Geometry: final body of the model. Coordinates: model frame, mm. A direction names the side the tool comes from. Round coordinates to 2 decimals unless told otherwise and drop trailing zeros. Write each loop counter-clockwise with the first axis right and the second up, starting at its lowest first coordinate (ties: lowest second). Pieces come first, ordered by that corner, then holes. Notation, with made-up numbers: M -15,-20.5 L 17,-20.5 A22 cw 17,-11.5 Z; hole C 62.25,87.5 d5. An arc over 180 degrees is marked long. Use one line per item in the form item = value. Start each with the question number.
Item 1: Section query A-A (z = 1.4). Return loops of the section in (x, y).
Item 2: Pin query (flat end, axial travel): pin 1 Ø2 at (x, y) = (5, -2.5) entering from +Z. Return the tip coordinate at first contact, or that it passes through.
Item 3: Section query C-C (x = 10). Return loops of the section in (y, z).
Item 4: Ray query, probe 1 along X at (y, z) = (0.25, 0.45); probe 2 along X at (y, z) = (-0.25, 1.35); probe 3 along Y at (x, z) = (22.5, 1.05). Return the intervals inside material, ascending.
Item 5: Pull-direction query (Y, two-part tool) for faces 1 (the flat face through (31, -1, 2)), 2 (the cylindrical face through (26.92, -0.4, 0.99)), 3 (the cylindrical face through (12.888, -0.368, 0.597)), 4 (the cylindrical face through (-0.92, -0.4, 1.01)); classes: pulls with the +Y half, pulls with the -Y half, needs draft (parallel to the pull), parting line crosses it, or undercut.
Item 6: Reachability of faces 5 (the cylindrical face through (23.465, -0.301, 1.715)), 6 (the cylindrical face through (23.535, -1.715, 1.699)), 7 (the cylindrical face through (2.465, -1.699, 0.285)) from +Z, -Z, +X, -X, +Y, -Y: full face, straight path, thin tool, end or side. Return the list, or none.
from build123d import *

# Parameters (mm, degrees)
EXTRUDE_1_DEPTH     = 2
SKETCH_3_R          = 0.75
EXTRUDE_2_DEPTH     = 20
SKETCH_6_R          = 2
CUT_EXTRUDE_1_DEPTH = 20
SKETCH_7_R          = 2
CUT_EXTRUDE_2_DEPTH = 20
FILLET_2_R          = 1
FILLET_3_R          = 1


with BuildPart() as part:
    # 草图2 → 凸台-拉伸1 (new body)
    with BuildSketch(Plane.XY):
        with BuildLine():
            Line((0, 0), (5, 0))
            Line((5, 0), (5, -2))
            Line((5, -2), (0, -2))
            ThreePointArc((0, -2), (-5.828427125, -1), (0, 0))
        make_face()
    extrude_1 = extrude(amount=EXTRUDE_1_DEPTH)

    # 草图3 → 凸台-拉伸2 (add)
    with BuildSketch(Plane(origin=(5, 0, 0), x_dir=(0, 0, -1), z_dir=(1, 0, 0))):
        with Locations((-1, -1)):
            Circle(SKETCH_3_R)
    extrude(amount=EXTRUDE_2_DEPTH)

    # 草图6 → 切除-拉伸1 (cut)
    with BuildSketch(Plane.XY.offset(2)):
        with Locations((-2.828427125, -1)):
            Circle(SKETCH_6_R)
    extrude(amount=-CUT_EXTRUDE_1_DEPTH, mode=Mode.SUBTRACT)

    # 镜向9: 凸台-拉伸1 across plane
    add(extrude_1.mirror(Plane(origin=(13, 0, 0), x_dir=(0, 0, 1), z_dir=(1, 0, 0))))

    # 草图7 → 切除-拉伸2 (cut)
    with BuildSketch(Plane(origin=(0, 0, 0), x_dir=(-1, 0, 0), z_dir=(0, 0, -1))):
        with Locations((-28.828427125, -1)):
            Circle(SKETCH_7_R)
    extrude(amount=-CUT_EXTRUDE_2_DEPTH, mode=Mode.SUBTRACT)

    # 圆角2
    fillet_2_edges = [part.edges().sort_by_distance(p)[0] for p in [
        (2.5, -2, 2),
        (2.5, -2, 0),
        (2.5, 0, 0),
        (2.5, 0, 2),
    ]]
    fillet(fillet_2_edges, radius=FILLET_2_R - 0.0001)  # a hair under: the kernel refuses the full size

    # 圆角3
    fillet_3_edges = [part.edges().sort_by_distance(p)[0] for p in [
        (23.5, -2, 2),
        (23.5, -2, 0),
        (23.5, 0, 0),
        (23.5, 0, 2),
    ]]
    fillet(fillet_3_edges, radius=FILLET_3_R - 0.0001)  # a hair under: the kernel refuses the full size


solid = part.part
Working result:
q1.outline = M 0.03,-1.92 L 5,-1.92 L 5,-1.63 L 21,-1.63 L 21,-1.92 L 25.97,-1.92 A3 ccw long 25.97,-0.08 L 21,-0.08 L 21,-0.37 L 5,-0.37 L 5,-0.08 L 0.03,-0.08 A3 ccw long Z; hole C -2.83,-1 d4; hole C 28.83,-1 d4
q2.pin_1 = 1.87
q3.outline = C -1,1 d1.5
q4.probe_1 = -5.56 to -4.39, -1.27 to -0.1, 26.1 to 27.27, 30.39 to 31.56
q4.probe_2 = -5.73 to -4.68, -0.97 to 5, 21 to 26.97, 30.68 to 31.73
q4.probe_3 = -2 to 0
q5.face_1 = needs draft
q5.face_2 = undercut
q5.face_3 = parting line crosses it
q5.face_4 = undercut
q6.face_5 = +Z, +Y
q6.face_6 = +Z, -Y
q6.face_7 = -Z, -Y
